Can you work these out from the drawing? Everything is in mm from the part's minimum corner. A direction names the side the tool comes from. Give positions to 0.01 mm unless a question says otherwise; leave off trailing zeros. Write each loop counter-clockwise with the first axis right and the second up, starting at its lowest first coordinate (ties: lowest second). Pieces come first, ordered by that corner, then holes. Notation, with made-up numbers: (57, -5.75) -> (78, -5.75) arc R11 cw to (78, 9.25) -> close; hole circle Ø9 at (88, 3). An arc over 180 degrees is marked (long way). Answer as CSV lines item,"result". Start each with the question number.
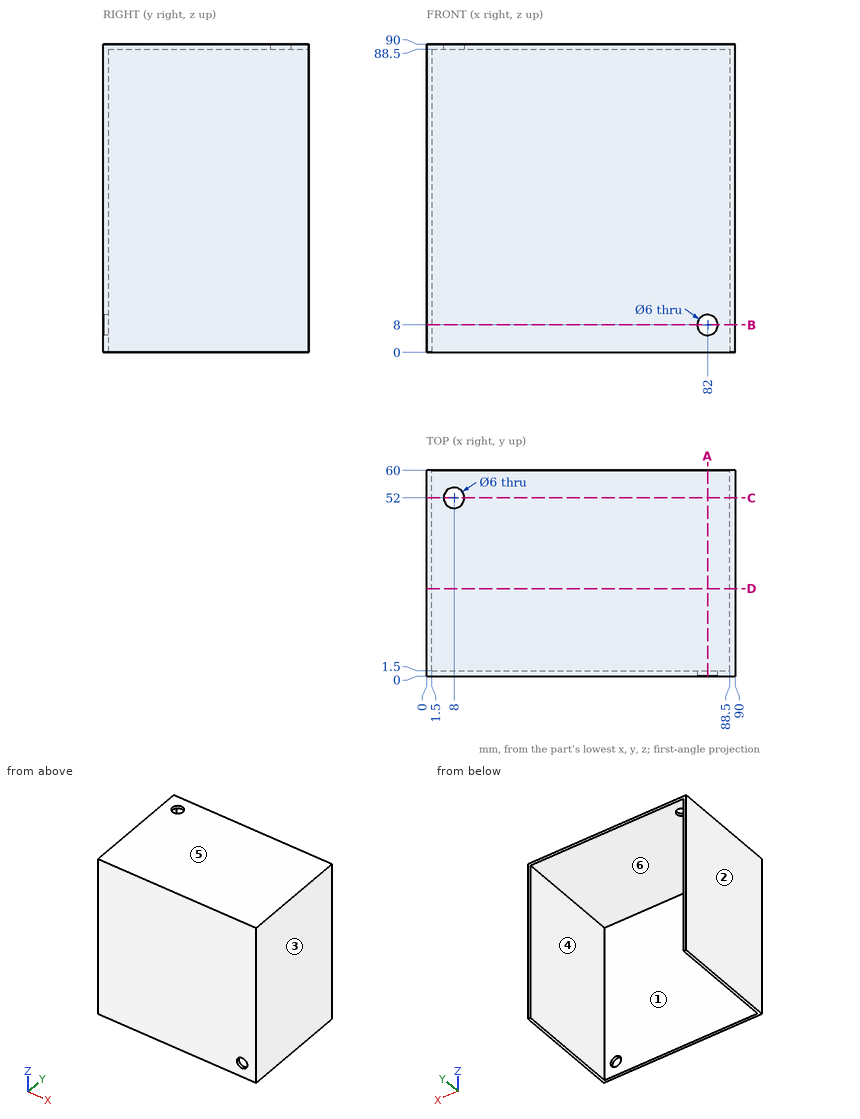
Item 1: If we section it at B-B (z = 8): Please give me the cut outline in (x, y), and give its area (4 significant figures).
Item 2: I'm going to push flat-ended pins straight in: pin 1 (5 mm diameter, centred on x = 32.5, y = 38, fed in from -Z); pin 2 (6 mm diameter, centred on x = 11.5, z = 66, fed in from +Y). Where does each tip first touch, or does it pass through?
Item 3: If we section it at C-C (y = 52): Please give me the cut outline in (x, z), and give its area (4 significant figures).
Item 4: We'd pull the mould along X, two halves only. Please class the marked faces 1, 2, 3 and 4: released by +X, released by -X, zero draft, split by the parting line, or undercut.
Item 5: If we section it at A-A (x = 82): Please give me the cut outline in (y, z), and give its area (3 significant figures).
Item 6: For the marked faces 5 and 6, which set-ups out of +Z, -Z, +X, -X, +Y, -Y let a thin tool reach every point of the face, with its end or its side?
Item 7: If we section it at D-D (y = 25.5): Please give me the cut outline in (x, z).
Item 8: If I drill on line 1 (X direction, y = 21, z = 37.5); line 2 (Y direction, x = 8, z = 89); line 3 (Z direction, x = 32, y = 42), over which ranges is the centre line in solid material (lowest first)? Write a range as [from, to].
Final values:
1,outline,"(0, 0) -> (79, 0) -> (79, 1.5) -> (1.5, 1.5) -> (1.5, 60) -> (0, 60) -> close; (85, 0) -> (90, 0) -> (90, 60) -> (88.5, 60) -> (88.5, 1.5) -> (85, 1.5) -> close"
1,area,"301.5 mm2"
2,pin 1,"z = 88.5"
2,pin 2,"y = 1.5"
3,outline,"(0, 0) -> (1.5, 0) -> (1.5, 88.5) -> (5, 88.5) -> (5, 90) -> (0, 90) -> close; (11, 88.5) -> (88.5, 88.5) -> (88.5, 0) -> (90, 0) -> (90, 90) -> (11, 90) -> close"
3,area,"391.5 mm2"
4,face 1,"undercut"
4,face 2,"released by -X"
4,face 3,"released by +X"
4,face 4,"undercut"
5,outline,"(0, 0) -> (1.5, 0) -> (1.5, 5) -> (0, 5) -> close; (0, 11) -> (1.5, 11) -> (1.5, 88.5) -> (60, 88.5) -> (60, 90) -> (0, 90) -> close"
5,area,"214 mm2"
6,face 5,"+Z, +X, -X, +Y, -Y"
6,face 6,"-Z, +Y"
7,outline,"(0, 0) -> (1.5, 0) -> (1.5, 88.5) -> (88.5, 88.5) -> (88.5, 0) -> (90, 0) -> (90, 90) -> (0, 90) -> close"
8,line 1,"[0, 1.5], [88.5, 90]"
8,line 2,"[0, 49], [55, 60]"
8,line 3,"[88.5, 90]"
